```python
from build123d import *

# Parameters (mm, degrees)
FILLET1_R = 1.5
FILLET2_R = 0.25


with BuildPart() as part:
    # Sketch2 → Revolve1 (revolve)
    with BuildSketch(Plane(origin=(0, 0, 0), x_dir=(0, 0, -1), z_dir=(1, 0, 0))):
        with BuildLine():
            Line((-90, 0), (10, 0))
            Line((10, 0), (10, 3))
            Line((10, 3), (0, 3))
            Line((0, 3), (0, 5))
            Line((0, 5), (-10, 5))
            ThreePointArc((-10, 5), (-14.152273993, 5.172712088), (-18.275862069, 5.689655172))
            ThreePointArc((-18.275862069, 5.689655172), (-29.100280769, 7.04663077), (-40, 7.5))
            Line((-40, 7.5), (-90, 7.5))
            Line((-90, 7.5), (-90, 0))
        make_face()
    revolve(axis=Axis((0, 0, -121.417180302), (0, 0, 1)))

    # Fillet1
    fillet1_edges = [part.edges().sort_by_distance(p)[0] for p in [
        (0, -7.5, 90),
    ]]
    fillet(fillet1_edges, radius=FILLET1_R)

    # Fillet2
    fillet2_edges = [part.edges().sort_by_distance(p)[0] for p in [
        (0, -5, 0),
    ]]
    fillet(fillet2_edges, radius=FILLET2_R)


solid = part.part
```
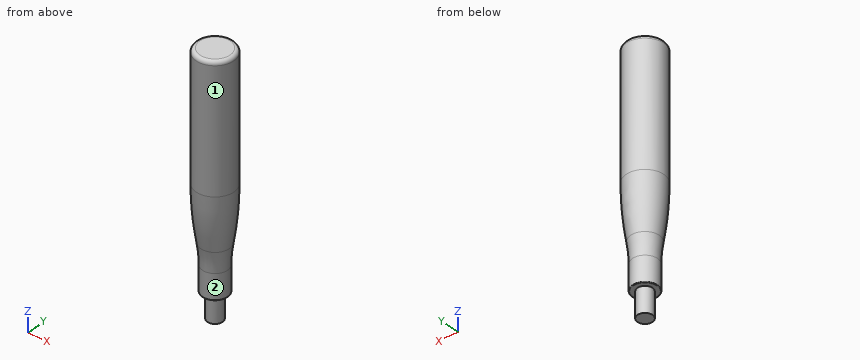
CAD build for the part. Positions are in the model's coordinates, mm. Face numbers are marked on the shaded views. A direction names the side the tool comes from. Round coordinates to 2 decimals unless told otherwise and drop trailing zeros. Order: outer loops, then holes, each group sorted by start corner. A loop starts at its lowest first (then second) coordinate and runs counter-clockwise, first axis right, second up. Notation, with made-up numbers: (83, 19) - (94, 19) arc R17 ccw to (94, 46) - close; hole circle Ø2 at (-13, 5). An arc over 180 degrees is marked (long way). Answer as CSV lines item,"result". Start each with the question number.
1. Pin check, flat tips, straight feed: pin 1 (6 mm diameter, centred on x = -4, y = 3.5, fed in from -Z); pin 2 (1 mm diameter, centred on y = -5, z = 60.5, fed in from +X). Stop position of each tip, or through.
2. Saw through at B-B, the plane z = -1.5. Write the cut outline in (x, y), and give its area (3 significant figures).
3. Tool access for the marked faces 1 and 2: list every direction of +Z, -Z, +X, -X, +Y, -Y with a clear straight run to the whole face (end or side of a thin tool).
4. Drill centre lines: L1, parallel to Z at x = 1, y = -3.75; L2, parallel to X at y = 4.5, z = 51.5; L3, parallel to X at y = 0.5, z = 74. Where is each one in solid material? Low to high. Write a range as [from, to].
5. Saw through at A-A, the plane z = 76. Write the cut outline in (x, y), and give its area (3 significant figures).
Model answer:
1,pin 1,"stops at z = -10"
1,pin 2,"stops at x = 6"
2,outline,"circle Ø6 at (0, 0)"
2,area,"28.3 mm²"
3,face 1,"+Z, -Z"
3,face 2,"-Z"
4,L1,"z = [0, 90]"
4,L2,"x = [-6, 6]"
4,L3,"x = [-7.48, 7.48]"
5,outline,"circle Ø15 at (0, 0)"
5,area,"177 mm²"
